from build123d import *

# Parameters (mm, degrees)
SKETCH1_W           = 1000
SKETCH1_H           = 1000
SKETCH1_W_2         = 800
SKETCH1_H_2         = 800
BOSS_EXTRUDE1_DEPTH = 1000
SKETCH2_R           = 205
BOSS_EXTRUDE2_DEPTH = 600


with BuildPart() as part:
    # Sketch1 → Boss-Extrude1 (new body)
    with BuildSketch(Plane.XY):
        with Locations((500, 500)):
            Rectangle(SKETCH1_W, SKETCH1_H)
        with Locations((500, 500)):
            Rectangle(SKETCH1_W_2, SKETCH1_H_2, mode=Mode.SUBTRACT)
    extrude(amount=BOSS_EXTRUDE1_DEPTH)

    # Sketch2 → Boss-Extrude2 (add)
    with BuildSketch(Plane.XZ.offset(-900)):
        with Locations(Location((500, 750, 0), (0, 0, 90))):
            Circle(SKETCH2_R)
    extrude(amount=BOSS_EXTRUDE2_DEPTH)


solid = part.part
For this review, take the finished solid that the model builds, in its own axes (mm). A direction names the side the tool comes from. Round coordinates to 2 decimals unless told otherwise and drop trailing zeros. Order: outer loops, then holes, each group sorted by start corner. A loop starts at its lowest first (then second) coordinate and runs counter-clockwise, first axis right, second up. Notation, with made-up numbers: M 20,24.5 L 64,24.5 A23 cw 64,46.5 Z; hole C 57,75 d8. An arc over 180 degrees is marked long. Use a Markdown table: item, result. Add a question column.
Item 1: Tool access review of faces 1 (the flat face through (0, 493, 493)), 2 (the cylindrical face through (578.516, 604.2, 939.368)), 3 (the flat face through (497, 300, 747)): name each direction out of +Z, -Z, +X, -X, +Y, -Y from which nothing blocks a thin tool from reaching the whole face with its end or side.
Item 2: Insertion check: pin 1 (10 mm diameter, centred on x = 440.5, y = 781, fed in from -Z); pin 2 (6 mm diameter, centred on x = 380.5, y = 602.5, fed in from -Z). Each pin has a flat end and moves straight along its axis. Give the tip position at first contact, or say it passes through.
Item 3: Add section D-D, the plane x = 500. Give the boundary of the cut face in (y, z), then the cut area to 3 significant figures.
Item 4: Add section B-B, the plane x = 835. Give the boundary of the cut face in (y, z).
Item 5: Add section C-C, the plane z = 750. Give the boundary of the cut face in (x, y), then the cut area to 3 significant figures.
Item 6: Mouldability with a two-part tool opening along Y and no side actions: class faces 4 (the flat face through (493, 1000, 493)), 5 (the flat face through (937, 507, 1000)), 6 (the flat face through (900, 494, 493)) as released by +Y, released by -Y, zero draft, split by the parting line, or undercut.
Item 7: To check wall thickness, follow line 1 along Y through (x, z) = (127, 683); line 2 along Y through (x, z) = (546, 612). State the ranges of each line that lie inside material, in increasing order.
Item 8: Add section A-A, the plane y = 638.5. Give the boundary of the cut face in (x, z), then the cut area to 3 significant figures.
Geometry results:
| question | item | result |
|---|---|---|
| 1 | face 1 | +Z, -Z, -X, +Y, -Y |
| 1 | face 2 | none |
| 1 | face 3 | +Z, -Z |
| 2 | pin 1 | stops at z = 552.38 |
| 2 | pin 2 | stops at z = 581.32 |
| 3 | outline | M 0,0 L 100,0 L 100,1000 L 0,1000 Z; M 300,545 L 900,545 L 900,0 L 1000,0 L 1000,1000 L 900,1000 L 900,955 L 300,955 Z |
| 3 | area | 446,000 mm² |
| 4 | outline | M 0,0 L 100,0 L 100,1000 L 0,1000 Z; M 900,0 L 1000,0 L 1000,1000 L 900,1000 Z |
| 5 | outline | M 0,0 L 1000,0 L 1000,1000 L 0,1000 Z; hole M 100,100 L 900,100 L 900,900 L 705,900 L 705,300 L 295,300 L 295,900 L 100,900 Z |
| 5 | area | 606,000 mm² |
| 6 | face 4 | released by +Y |
| 6 | face 5 | zero draft |
| 6 | face 6 | undercut |
| 7 | line 1 | y = 0 to 100, 900 to 1000 |
| 7 | line 2 | y = 0 to 100, 300 to 1000 |
| 8 | outline | M 0,0 L 100,0 L 100,1000 L 0,1000 Z; C 500,750 d410; M 900,0 L 1000,0 L 1000,1000 L 900,1000 Z |
| 8 | area | 332,000 mm² |
